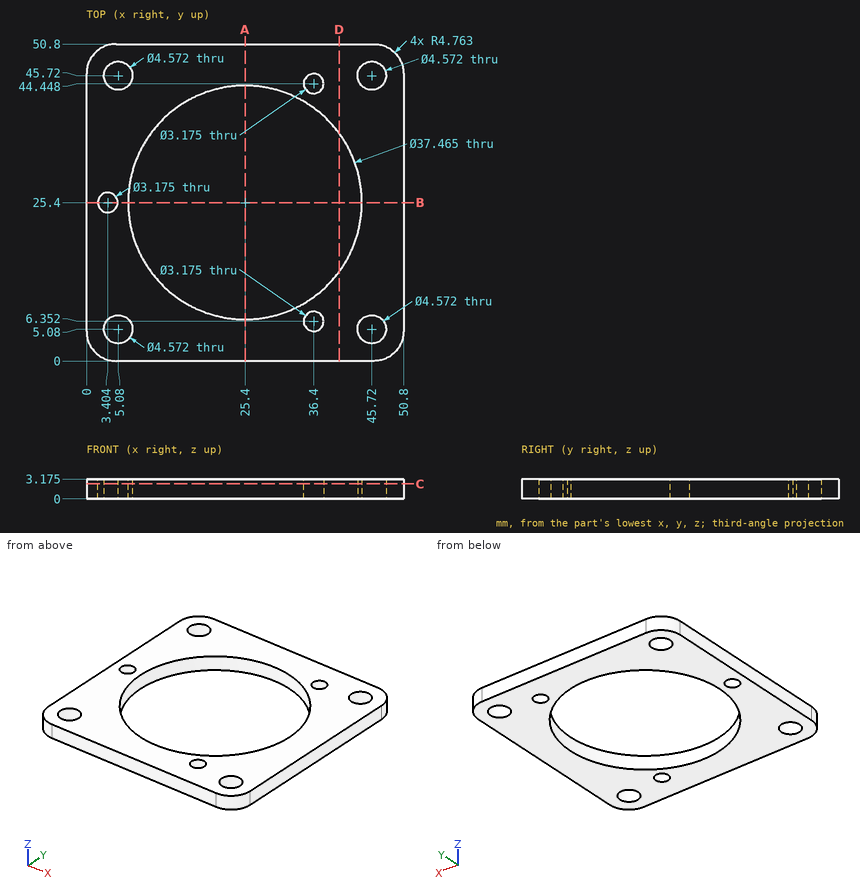
The figure shows three views and two pictorial views of one solid part (mm, origin at its lowest corner). Answer the questions. Give positions to 0.01 mm unless a question says otherwise; leave off trailing zeros. Write each loop counter-clockwise with the first axis right and the second up, starting at its lowest first coordinate (ties: lowest second). Pieces come first, ordered by that corner, then holes. Notation, with made-up numbers: M 85,-0.5 L 89,-0.5 A24 ccw 89,35.5 Z; hole C -37,62.5 d2. An arc over 180 degrees is marked long. One line per item, written item: value. Start each with the question number.
(1) Find section A-A (x = 25.4). Determine the outline of the cut face in (y, z) (1 decimal).
(2) Find section B-B (y = 25.4). Determine the outline of the cut face in (x, z) (1 decimal).
(3) Find section C-C (z = 2.4). Give the number of separate pieces and of enclosed holes in the cut face, plus the area to 3 significant figures.
(4) Find section D-D (x = 40.5). Determine the outline of the cut face in (y, z) (1 decimal).
(5) Find the intervals of material crossed by line 1 (Y direction, x = 45.72, z = 1.1) (1 decimal); line 2 (Y direction, x = 26, z = 0.95); line 3 (X direction, y = 4.5, z = 3), in increasing order.
Results below:
1. outline: M 0,0 L 6.7,0 L 6.7,3.2 L 0,3.2 Z; M 44.1,0 L 50.8,0 L 50.8,3.2 L 44.1,3.2 Z
2. outline: M 0,0 L 1.8,0 L 1.8,3.2 L 0,3.2 Z; M 5,0 L 6.7,0 L 6.7,3.2 L 5,3.2 Z; M 44.1,0 L 50.8,0 L 50.8,3.2 L 44.1,3.2 Z
3. separate pieces: 1
3. enclosed holes: 8
3. area: 1,370 mm^2
4. outline: M 0,0 L 14.3,0 L 14.3,3.2 L 0,3.2 Z; M 36.5,0 L 50.8,0 L 50.8,3.2 L 36.5,3.2 Z
5. line 1: y = 0 to 2.8, 7.4 to 43.4, 48 to 50.8
5. line 2: y = 0 to 6.68, 44.12 to 50.8
5. line 3: x = 0.01 to 2.87, 7.29 to 43.51, 47.93 to 50.79
